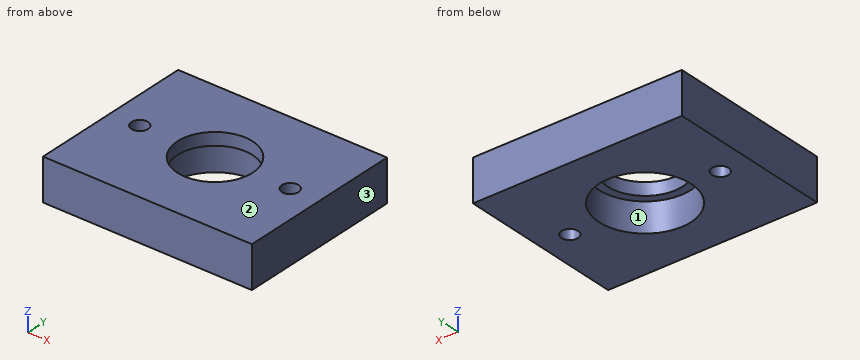
from build123d import *

# Parameters (mm, degrees)
SKETCH1_W           = 50
SKETCH1_H           = 40
SKETCH1_R           = 11
SKETCH1_R_2         = 2
BOSS_EXTRUDE1_DEPTH = 10
SKETCH2_R           = 11
SKETCH2_R_2         = 9
BOSS_EXTRUDE2_DEPTH = 3


with BuildPart() as part:
    # Sketch1 → Boss-Extrude1 (new body)
    with BuildSketch(Plane.XY):
        Rectangle(SKETCH1_W, SKETCH1_H)
        Circle(SKETCH1_R, mode=Mode.SUBTRACT)
        with Locations((-18, 0)):
            Circle(SKETCH1_R_2, mode=Mode.SUBTRACT)
        with Locations((18, 0)):
            Circle(SKETCH1_R_2, mode=Mode.SUBTRACT)
    extrude(amount=BOSS_EXTRUDE1_DEPTH)

    # Sketch2 → Boss-Extrude2 (add)
    with BuildSketch(Plane.XY.offset(10)):
        Circle(SKETCH2_R)
        Circle(SKETCH2_R_2, mode=Mode.SUBTRACT)
    extrude(amount=-BOSS_EXTRUDE2_DEPTH)


solid = part.part
Work out the finished part from the listing and answer in its coordinate system (mm). Face numbers are marked on the shaded views. Give positions to 0.01 mm unless a question says otherwise; leave off trailing zeros. Loops run counter-clockwise (first coordinate to the right, second up) from the corner with the lowest first, then second, coordinate; pieces in that order, holes last. Notation, with made-up numbers: (62, -15) -> (91, -15) arc R25 cw to (91, 17) -> close; hole circle Ø10 at (75.25, -26.5). An arc over 180 degrees is marked (long way). Use a Markdown table: item, result. Add a question column.
1) For a pull along X with two mould halves and no side action, classify the marked faces 1, 2 and 3 as +X half, -X half, draft (parallel to the pull), parting line (faces both ways), or undercut.
2) This flat-tipped pin is pushed along its axis until it touches: P1, Ø20.5, axis at x = 0, y = 0, coming from the -Z side. Where does it stop, or does it pass through?
3) The part is cut by section B-B, the plane z = 3. Determine the outline of the cut face in (x, y).
4) The part is cut by section D-D, the plane y = -10. Determine the outline of the cut face in (x, z), plus the area to 3 significant figures.
5) The part is cut by section A-A, the plane x = -18. Determine the outline of the cut face in (y, z), plus the area to 3 significant figures.
6) Consider line 1 along Y through (x, z) = (0, 2.5); line 2 along Y through (x, z) = (0, 8.35); line 3 along Z through (x, y) = (5.5, -7.5). Determine where each line is inside the solid, lowest interval first.
7) The part is cut by section C-C, the plane x = 0. Determine the outline of the cut face in (y, z).
Reported:
| question | item | result |
|---|---|---|
| 1 | face 1 | undercut |
| 1 | face 2 | draft |
| 1 | face 3 | +X half |
| 2 | P1 | stops at z = 7 |
| 3 | outline | (-25, -20) -> (25, -20) -> (25, 20) -> (-25, 20) -> close; hole circle Ø4 at (-18, 0); hole circle Ø22 at (0, 0); hole circle Ø4 at (18, 0) |
| 4 | outline | (-25, 0) -> (-4.58, 0) -> (-4.58, 7) -> (4.58, 7) -> (4.58, 0) -> (25, 0) -> (25, 10) -> (-25, 10) -> close |
| 4 | area | 436 mm^2 |
| 5 | outline | (-20, 0) -> (-2, 0) -> (-2, 10) -> (-20, 10) -> close; (2, 0) -> (20, 0) -> (20, 10) -> (2, 10) -> close |
| 5 | area | 360 mm^2 |
| 6 | line 1 | y = -20 to -11, 11 to 20 |
| 6 | line 2 | y = -20 to -9, 9 to 20 |
| 6 | line 3 | z = 7 to 10 |
| 7 | outline | (-20, 0) -> (-11, 0) -> (-11, 7) -> (-9, 7) -> (-9, 10) -> (-20, 10) -> close; (9, 7) -> (11, 7) -> (11, 0) -> (20, 0) -> (20, 10) -> (9, 10) -> close |
